```python
from build123d import *

# Parameters (mm, degrees)
F1_DEPTH = 63.5
F2_DEPTH = 25.4
F3_DEPTH = 7.9375
F4_DEPTH = 25.4


with BuildPart() as f1:
    # F0 (on Front) → F1 (new body, symmetric)
    with BuildSketch(Plane.XZ):
        Polygon((-41.275, 9.525), (-41.275, -9.525), (41.275, -9.525), (41.275, 9.525), (31.566352, 9.525), align=None)
    extrude(amount=F1_DEPTH, both=True)

    # F0 (on Front) → F2 (join, symmetric)
    with BuildSketch(Plane.XZ):
        with BuildLine():
            Line((31.566352, 9.525), (41.275, 9.525))
            Line((41.275, 9.525), (41.275, 41.2877))
            ThreePointArc((41.275, 41.2877), (45.92468, 52.51302), (57.15, 57.1627))
            Line((57.15, 57.1627), (68.645397, 57.1627))
            Line((68.645397, 57.1627), (68.645397, 66.871348))
            Line((68.645397, 66.871348), (57.15, 66.871348))
            add(Edge.make_bspline(
                [(55.419964, 66.812786), (55.99465, 66.83655), (56.571327, 66.856085), (57.15, 66.871348)],
                knots=[112.39165, 112.39165, 112.39165, 112.39165, 113.912617, 113.912617, 113.912617, 113.912617], degree=3))
            ThreePointArc((55.419964, 66.812786), (38.457974, 58.755705), (31.566352, 41.2877))
            Line((31.566352, 41.2877), (31.566352, 9.525))
        make_face()
    extrude(amount=F2_DEPTH, both=True)

    # F0 (on Front) → F3 (join, symmetric)
    with BuildSketch(Plane.XZ):
        with BuildLine():
            add(Edge.make_bspline(
                [(-41.275, 9.525), (-18.64041, 40.209658), (12.953615, 65.056772), (55.419964, 66.812786)],
                knots=[0, 0, 0, 0, 112.39165, 112.39165, 112.39165, 112.39165], degree=3))
            Line((-41.275, 9.525), (31.566352, 9.525))
            Line((31.566352, 9.525), (31.566352, 41.2877))
            ThreePointArc((31.566352, 41.2877), (38.457974, 58.755705), (55.419964, 66.812786))
        make_face()
    extrude(amount=F3_DEPTH, both=True)

    # F0 (on Front) → F4 (join, symmetric)
    with BuildSketch(Plane.XZ):
        Polygon((68.645397, 71.4502), (68.645397, 66.871348), (68.645397, 57.1627), (68.645397, 42.8752), (85.446604, 42.8752), (84.830329, 71.4502), align=None)
        Polygon((94.045397, 71.4502), (84.830329, 71.4502), (85.446604, 42.8752), (94.045397, 42.8752), (94.045397, 57.1627), align=None)
    extrude(amount=F4_DEPTH, both=True)


solid = f1.part
```
Can you work these out from the model? Positions are in its coordinate system, mm. A direction names the side the tool comes from. Give positions to 0.01 mm unless a question says otherwise; leave off trailing zeros. Order: outer loops, then holes, each group sorted by start corner. A loop starts at its lowest first (then second) coordinate and runs counter-clockwise, first axis right, second up. Notation, with made-up numbers: M 70.25,-23.75 L 97.25,-23.75 A29 ccw 97.25,2.25 Z; hole C 9,85 d10. An arc over 180 degrees is marked long. One line per item, written item: value.
1) I want a section at A-A, the plane x = 62.5. List the corners of the cut face in (y, z) for me, plus the area to 3 significant figures.
Answer sheet:
outline: M -25.4,57.16 L 25.4,57.16 L 25.4,66.87 L -25.4,66.87 Z
area: 493 mm^2
2) I want a section at B-B, the plane y = 35.5. List the corners of the cut face in (x, z) for me (3 decimals), plus the area to 3 significant figures.
Answer sheet:
outline: M -41.275,-9.525 L 41.275,-9.525 L 41.275,9.525 L -41.275,9.525 Z
area: 1,570 mm^2
3) Please list where these lines run through material, in increasing order: line 1 along Y through (x, z) = (3, 17); line 2 along Z through (x, y) = (-30, -10) (3 decimals); line 3 along X through (y, z) = (13, 11.5) (3 decimals).
Answer sheet:
line 1: y = -7.94 to 7.94
line 2: z = -9.525 to 9.525
line 3: x = 31.566 to 41.275
4) For P1, Ø4.5, axis at y = -4.5, z = 52.5, coming from the -X side; P2, Ø6, axis at x = 19, z = 25.5, coming from the -Y side; P3, Ø6, axis at x = 64, y = 17.5, coming from the -Z side, each with a flat end and sliding along its axis, tell me the tip position at first contact or that it passes through.
Answer sheet:
P1: stops at x = 1.6
P2: stops at y = -7.94
P3: stops at z = 57.16
5) We'd pull the mould along X, two halves only. Please class faces 1 (the face through (68.645, 0, 50)), 2 (the face through (70, -25.4, 48)), 3 (the face through (63, 0, 57.163)), 4 (the face through (38.64, -16.79, 58.95)): released by +X, released by -X, zero draft, split by the parting line, or undercut.
Answer sheet:
face 1: undercut
face 2: zero draft
face 3: undercut
face 4: released by -X
6) On a 3-axis mill with a long thin cutter (end or side, diameter ignored), from which of +Z, -Z, +X, -X, +Y, -Y can I reach the whole of each face in a straight line? I mean faces 5 (the face through (45.802, -0.356, 52.389)), 6 (the face through (70, 25.4, 48)), 7 (the face through (8, -7.938, 32)), 8 (the face through (63, 0, 66.871)). Say none if no direction works.
Answer sheet:
face 5: -Z, +Y, -Y
face 6: +Z, +X, -X, +Y
face 7: +Z, -X, -Y
face 8: +Z, -X, +Y, -Y
